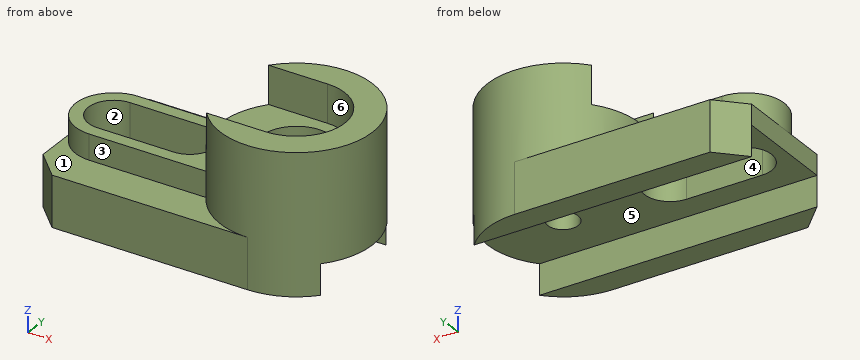
```python
from build123d import *

# Parameters (mm, degrees)
ESBO_O3_R                = 30
RESSALTO_EXTRUS_O1_DEPTH = 55
RESSALTO_EXTRUS_O2_START = -20
RESSALTO_EXTRUS_O2_DEPTH = 20
CORTE_EXTRUS_O2_DEPTH    = 15
ESBO_O9_R                = 14
CORTE_EXTRUS_O6_DEPTH    = 5
ESBO_O12_R               = 6
CORTE_EXTRUS_O7_DEPTH    = 65
CHANFRO2_SIZE            = 10
CHANFRO3_SIZE            = 10
RESSALTO_EXTRUS_O4_START = 10
RESSALTO_EXTRUS_O4_DEPTH = 10
CORTE_EXTRUS_O8_DEPTH    = 54
ESBO_O16_W               = 12
ESBO_O16_H               = 40
CORTE_EXTRUS_O9_DEPTH    = 124


with BuildPart() as part:
    # Esboço3 → Ressalto-extrusão1 (new body)
    with BuildSketch(Plane.XY):
        Circle(ESBO_O3_R)
    extrude(amount=-RESSALTO_EXTRUS_O1_DEPTH)

    # Esboço4 → Ressalto-extrusão2 (add)
    with BuildSketch(Plane(origin=(0, 0, -55), x_dir=(-1, 0, 0), z_dir=(0, 0, -1)).offset(RESSALTO_EXTRUS_O2_START)):
        with BuildLine():
            Line((0, 30), (87, 30))
            Line((87, 30), (87, -30))
            Line((87, -30), (0, -30))
            ThreePointArc((0, -30), (30, 0), (0, 30))
        make_face()
    extrude(amount=RESSALTO_EXTRUS_O2_DEPTH)

    # Esboço6 → Corte-extrusão2 (cut)
    with BuildSketch(Plane.XY):
        with BuildLine():
            Line((0, -19), (-43.25121435, -19))
            Line((-43.25121435, -19), (-43.25121435, 19))
            Line((-43.25121435, 19), (0, 19))
            ThreePointArc((0, 19), (19, 0), (0, -19))
        make_face()
    extrude(amount=-CORTE_EXTRUS_O2_DEPTH, mode=Mode.SUBTRACT)

    # Esboço9 → Corte-extrusão6 (cut)
    with BuildSketch(Plane.XY.offset(-15)):
        Circle(ESBO_O9_R)
    extrude(amount=-CORTE_EXTRUS_O6_DEPTH, mode=Mode.SUBTRACT)

    # Esboço12 → Corte-extrusão7 (cut)
    with BuildSketch(Plane.XY.offset(-20)):
        with Locations((0.167448048, 0.04248466)):
            Circle(ESBO_O12_R)
    extrude(amount=-CORTE_EXTRUS_O7_DEPTH, mode=Mode.SUBTRACT)

    # Chanfro2
    chanfro2_edges = [part.edges().sort_by_distance(p)[0] for p in [
        (-87, 30, -45),
    ]]
    chamfer(chanfro2_edges, length=CHANFRO2_SIZE)

    # Chanfro3
    chanfro3_edges = [part.edges().sort_by_distance(p)[0] for p in [
        (-87, -30, -45),
    ]]
    chamfer(chanfro3_edges, length=CHANFRO3_SIZE)

    # Esboço14 → Ressalto-extrusão4 (add)
    with BuildSketch(Plane.XY.offset(-35).offset(RESSALTO_EXTRUS_O4_START)):
        with BuildLine():
            Line((-72, 15), (-25.980762114, 15))
            ThreePointArc((-25.980762114, 15), (-30, 0), (-25.980762114, -15))
            Line((-25.980762114, -15), (-72, -15))
            ThreePointArc((-72, -15), (-87, 0), (-72, 15))
        make_face()
    extrude(amount=-RESSALTO_EXTRUS_O4_DEPTH)

    # Esboço15 → Corte-extrusão8 (cut)
    with BuildSketch(Plane.XY.offset(-25)):
        with BuildLine():
            Line((-72, 10), (-42, 10))
            ThreePointArc((-42, 10), (-32, 0), (-42, -10))
            Line((-42, -10), (-72, -10))
            ThreePointArc((-72, -10), (-82, 0), (-72, 10))
        make_face()
    extrude(amount=-CORTE_EXTRUS_O8_DEPTH, mode=Mode.SUBTRACT)

    # Esboço16 → Corte-extrusão9 (cut)
    with BuildSketch(Plane.ZY.offset(87)):
        with Locations((-49, 0)):
            Rectangle(ESBO_O16_W, ESBO_O16_H)
    extrude(amount=-CORTE_EXTRUS_O9_DEPTH, mode=Mode.SUBTRACT)


solid = part.part
```
CAD build for the part. Positions are in the model's coordinates, mm. Face numbers are marked on the shaded views. A direction names the side the tool comes from. Give positions to 0.01 mm unless a question says otherwise; leave off trailing zeros. Write each loop counter-clockwise with the first axis right and the second up, starting at its lowest first coordinate (ties: lowest second). Pieces come first, ordered by that corner, then holes. Notation, with made-up numbers: (57.5, 15.25) -> (111.5, 15.25) arc R22 cw to (111.5, 23.25) -> close; hole circle Ø4 at (74, 67). An arc over 180 degrees is marked (long way). Write each question's results on one line, items separated by ' | '.
1. Two-plate mould, pull along Y, no slides. Class the marked faces 1, 2 and 3: pulls with the +Y half, pulls with the -Y half, needs draft (parallel to the pull), parting line crosses it, or undercut.
Geometry check:
face 1: needs draft | face 2: undercut | face 3: pulls with the -Y half
2. Wall check: probe 1 along Y at (x, z) = (0, -18); probe 2 along Y at (x, z) = (-12.5, -47); probe 3 along X at (y, z) = (-2, -37.5). Give the ranges that are in metal, low to high. Write a range as [from, to].
Geometry check:
probe 1: [-30, -14], [14, 30] | probe 2: [-30, -20], [20, 30] | probe 3: [-87, -81.8], [-32.2, -5.47], [5.81, 29.93]
3. Which spindle directions (+Z, -Z, +X, -X, +Y, -Y) get a long thin tool onto all of the face, cutting with end or side? Do the marked faces 4, 5 and 6. Say none if no direction does.
Geometry check:
face 4: +Z, -Z | face 5: -Z, +X, -X | face 6: +Z, -X
4. Cut at D-D, the plane y = -25. Write the cut outline in (x, z), then the cut area to 3 significant figures.
Geometry check:
outline: (-82, -55) -> (16.58, -55) -> (16.58, 0) -> (-16.58, 0) -> (-16.58, -35) -> (-82, -35) -> close | area: 3,130 mm²
5. Cut at B-B, the plane y = -1.5. Write the cut outline in (x, z), then the cut area to 3 significant figures.
Geometry check:
outline: (-87, -43) -> (-81.89, -43) -> (-81.89, -25) -> (-86.92, -25) -> (-86.92, -35) -> (-87, -35) -> close; (-32.11, -43) -> (-5.63, -43) -> (-5.63, -20) -> (-13.92, -20) -> (-13.92, -15) -> (-29.96, -15) -> (-29.96, -25) -> (-32.11, -25) -> close; (5.97, -43) -> (29.96, -43) -> (29.96, 0) -> (18.94, 0) -> (18.94, -15) -> (13.92, -15) -> (13.92, -20) -> (5.97, -20) -> close | area: 1,570 mm²
6. Cut at C-C, the plane z = -33. Write the cut outline in (x, y).
Geometry check:
outline: (-72, -15) -> (-25.98, -15) arc R30 ccw (long way) to (-25.98, 15) -> (-72, 15) arc R15 ccw to start; hole (-72, -10) -> (-42, -10) arc R10 ccw to (-42, 10) -> (-72, 10) arc R10 ccw to start; hole circle Ø12 at (0.17, 0.04)
7. Drop flat-ended pins along their axis: P1, Ø1, axis at y = -22.5, z = -48, coming from the -X side; P2, Ø4, axis at x = -38, y = -17.5, coming from the +Z side; P3, Ø1.5, axis at x = -53.5, z = -32.5, coming from the +Y side. Give the stop position or say it passes through.
Geometry check:
P1: x = -85 | P2: z = -35 | P3: y = 15
8. Cut at A-A, the plane x = -56.5. Write the cut outline in (y, z), then the cut area to 3 significant figures.
Geometry check:
outline: (-30, -55) -> (-20, -55) -> (-20, -43) -> (-10, -43) -> (-10, -25) -> (-15, -25) -> (-15, -35) -> (-30, -35) -> close; (10, -43) -> (20, -43) -> (20, -55) -> (30, -55) -> (30, -35) -> (15, -35) -> (15, -25) -> (10, -25) -> close | area: 660 mm²
